from build123d import *

# Parameters (mm, degrees)
DODANIE_WYCI_GNI_CIE1_DEPTH = 5
SZKIC2_R                    = 2.2
WYTNIJ_WYCI_GNI_CIE1_DEPTH  = 10
SZKIC6_R                    = 2.5
WYTNIJ_WYCI_GNI_CIE3_DEPTH  = 163.864974749


with BuildPart() as part:
    # Szkic1 → Dodanie-wyciągnięcie1 (new body)
    with BuildSketch(Plane.XY):
        Polygon((0, -10), (-20, -10), (-20, -30), (160, -30), (160, -10), (140, -10), (140, 0), (0, 0), align=None)
    extrude(amount=DODANIE_WYCI_GNI_CIE1_DEPTH)

    # Szkic2 → Wytnij-wyciągnięcie1 (cut)
    with BuildSketch(Plane.XY.offset(5)):
        with Locations((35, -5)):
            Circle(SZKIC2_R)
        with Locations((105, -5)):
            Circle(SZKIC2_R)
    extrude(amount=-WYTNIJ_WYCI_GNI_CIE1_DEPTH, mode=Mode.SUBTRACT)

    # Szkic6 → Wytnij-wyciągnięcie3 (cut, through all)
    with BuildSketch(Plane.XY.offset(5)):
        with Locations((70, -20)):
            Circle(SZKIC6_R)
    extrude(amount=-WYTNIJ_WYCI_GNI_CIE3_DEPTH, mode=Mode.SUBTRACT)


solid = part.part
Can you work these out from the model? Positions are in its coordinate system, mm. A direction names the side the tool comes from. Coordinates: 2 decimals unless noted, no trailing zeros. Loops run counter-clockwise (first coordinate to the right, second up) from the corner with the lowest first, then second, coordinate; pieces in that order, holes last. Notation, with made-up numbers: (15, 45) - (34, 45) arc R19 cw to (34, 49) - close; hole circle Ø5 at (45, -16.75). An arc over 180 degrees is marked (long way). Put each result on its own line as item: value. Start each with the question number.
Item 1: Suppose I cut it at B-B (y = -20). Please give me the cut outline in (x, z).
Item 2: If we mould it in two halves opening along X, with no side actions, what happens to faces 4 (the face through (102.802, -4.903, 2.535)), 5 (the face through (0, -5, 2)), 6 (the face through (69, -15, 5))? For each: +X half, -X half, draft (parallel to the pull), parting line (faces both ways), or undercut.
Item 3: Suppose I cut it at D-D (y = -5). Please give me the cut outline in (x, z), and give its area (3 significant figures).
Item 4: If I drill on line 1 along Y through (x, z) = (70, 3.2); line 2 along X through (y, z) = (-19.75, 0.35); line 3 along X through (y, z) = (-6, 0.3), over which ranges is the centre line in solid material (lowest first)?
Item 5: Suppose I cut it at A-A (x = 70). Please give me the cut outline in (y, z).
Item 6: For pin 1 (2 mm diameter, centred on y = -6, z = 1.5, fed in from -X); pin 2 (2.5 mm diameter, centred on x = 155, z = 2, fed in from +Y); pin 3 (12 mm diameter, centred on x = 87, y = -8, fed in from -Z); pin 4 (1.5 mm diameter, centred on y = -6.5, z = 2.5, fed in from +X), each with a flat end and sliding along its axis, tell me the tip position at first contact or that it passes through.
Item 7: Which directions (+Z, -Z, +X, -X, +Y, -Y) give clear straight access to the entire face, cutting with the end or side of a thin tool? Please do faces 1 (the face through (140, -5, 2)), 2 (the face through (69, -30, 2)), 3 (the face through (-10, -10, 2)).
Item 8: Suppose I cut it at C-C (z = 3.2). Please give me the cut outline in (x, y), and give its area (3 significant figures).
Here are the results:
1. outline: (-20, 0) - (67.5, 0) - (67.5, 5) - (-20, 5) - close; (72.5, 0) - (160, 0) - (160, 5) - (72.5, 5) - close
2. face 4: undercut
2. face 5: -X half
2. face 6: draft
3. outline: (0, 0) - (32.8, 0) - (32.8, 5) - (0, 5) - close; (37.2, 0) - (102.8, 0) - (102.8, 5) - (37.2, 5) - close; (107.2, 0) - (140, 0) - (140, 5) - (107.2, 5) - close
3. area: 656 mm²
4. line 1: -30 to -22.5, -17.5 to 0
4. line 2: -20 to 67.51, 72.49 to 160
4. line 3: 0 to 33.04, 36.96 to 103.04, 106.96 to 140
5. outline: (-30, 0) - (-22.5, 0) - (-22.5, 5) - (-30, 5) - close; (-17.5, 0) - (0, 0) - (0, 5) - (-17.5, 5) - close
6. pin 1: x = 0
6. pin 2: y = -10
6. pin 3: z = 0
6. pin 4: x = 140
7. face 1: +Z, -Z, +X, +Y
7. face 2: +Z, -Z, +X, -X, -Y
7. face 3: +Z, -Z, -X, +Y
8. outline: (-20, -30) - (160, -30) - (160, -10) - (140, -10) - (140, 0) - (0, 0) - (0, -10) - (-20, -10) - close; hole circle Ø4.4 at (35, -5); hole circle Ø5 at (70, -20); hole circle Ø4.4 at (105, -5)
8. area: 4,950 mm²
